The drawing under review shows one solid part. Ordinate dimensions are in mm from its lowest x, y, z. Round coordinates to 2 decimals unless told otherwise and drop trailing zeros. Order: outer loops, then holes, each group sorted by start corner. A loop starts at its lowest first (then second) coordinate and runs counter-clockwise, first axis right, second up.
1) Mouldability with a two-part tool opening along X and no side actions: class the marked faces 1, 2, 3 and 4 as pulls with the +X half, pulls with the -X half, needs draft (parallel to the pull), parting line crosses it, or undercut.
2) Consider section B-B (y = 16). Give the boundary of the cut face in (x, z).
3) To check wall thickness, follow L1, parallel to Y at x = 13.5, z = 3.5; L2, parallel to X at y = 39, z = 3; L3, parallel to Z at x = 7.25, y = 52. State the ranges of each line that lie inside material, in increasing order.
4) Consider section A-A (x = 7.25). Give the boundary of the cut face in (y, z), then the cut area to 3 significant figures.
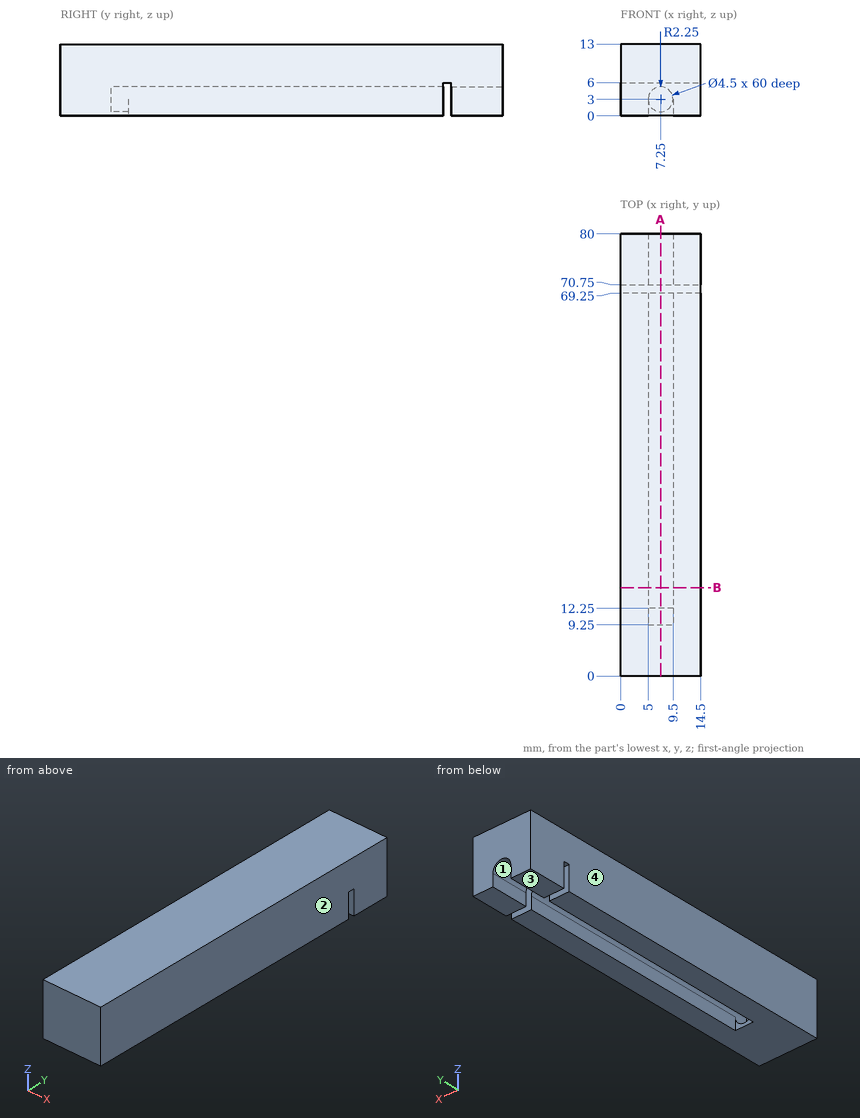
Answer below:
1. face 1: undercut
1. face 2: pulls with the +X half
1. face 3: needs draft
1. face 4: pulls with the -X half
2. outline: (0, 0) - (5, 0) - (5, 3) arc R2.25 cw to (9.5, 3) - (9.5, 0) - (14.5, 0) - (14.5, 13) - (0, 13) - close
3. L1: y = 0 to 69.25, 70.75 to 80
3. L2: x = 0 to 5, 9.5 to 14.5
3. L3: z = 5.25 to 13
4. outline: (0, 0) - (12.25, 0) - (12.25, 0.75) - (9.25, 0.75) - (9.25, 5.25) - (69.25, 5.25) - (69.25, 6) - (70.75, 6) - (70.75, 5.25) - (80, 5.25) - (80, 13) - (0, 13) - close
4. area: 670 mm2
